CAD build for the part. Positions are in the model's coordinates, mm. Coordinates: 2 decimals unless noted, no trailing zeros. Order: outer loops, then holes, each group sorted by start corner. A loop starts at its lowest first (then second) coordinate and runs counter-clockwise, first axis right, second up. Notation, with made-up numbers: M 69.5,-3.5 L 74.5,-3.5 A18 cw 74.5,5.5 Z; hole C -6,35 d1. An arc over 180 degrees is marked long. One line per item, written item: value.
from build123d import *

# Parameters (mm, degrees)
F1_DEPTH = 38.1
F2_R     = 25.4
F2_R_2   = 2.413
F3_DEPTH = 25.4
F4_R     = 3.429
F5_DEPTH = 25.4


with BuildPart() as f1:
    # F0 (on Right) → F1 (new body, symmetric)
    with BuildSketch(Plane.YZ):
        with BuildLine():
            ThreePointArc((5.6640261054, -4.752682216), (1.7239069957, -3.6969304825), (0, 0))
            Line((0, 0), (0, 76.2))
            Line((0, 76.2), (-3.175, 76.2))
            Line((-3.175, 76.2), (-3.175, 0))
            ThreePointArc((-3.175, 0), (-0.3169436651, -6.1291215894), (6.2153590695, -7.8794468319))
            Line((6.2153590695, -7.8794468319), (35.9767941298, -2.6317028461))
            Line((35.9767941298, -2.6317028461), (35.4254611657, 0.4950617697))
            Line((35.4254611657, 0.4950617697), (5.6640261054, -4.752682216))
        make_face()
    extrude(amount=F1_DEPTH, both=True)

    # F2 (on face) → F3 (cut)
    with BuildSketch(Plane.XZ.offset(3.175)):
        with Locations((0, 38.1)):
            Circle(F2_R)
        with Locations((-26.8363952125, 22.606)):
            Circle(F2_R_2)
        with Locations((0, 69.088)):
            Circle(F2_R_2)
        with Locations((26.8363952125, 22.606)):
            Circle(F2_R_2)
    extrude(amount=-F3_DEPTH, mode=Mode.SUBTRACT)

    # F4 (on face) → F5 (cut)
    with BuildSketch(Plane(origin=(0, 0.9835478115, -5.5779768219), x_dir=(1, 0, 0), z_dir=(0, -0.1736481777, 0.984807753))):
        with Locations((19.05, 15.9232353842)):
            Circle(F4_R)
        with Locations((-19.05, 15.9232353842)):
            Circle(F4_R)
    extrude(amount=-F5_DEPTH, mode=Mode.SUBTRACT)


solid = f1.part
Q1. Pin check, flat tips, straight feed: pin 1 Ø6 at (x, y) = (29.5, 13.5) entering from -Z; pin 2 Ø5.5 at (x, z) = (-26.84, 22.61) entering from +Y; pin 3 Ø4 at (x, z) = (0, 69.088) entering from -Y; pin 4 Ø1.5 at (x, y) = (-3.5, 9) entering from -Z. Stop position of each tip, or through.
Recorded:
pin 1: stops at z = -7.12
pin 2: stops at y = 0
pin 3: passes through
pin 4: stops at z = -7.52
Q2. Mould opens along Y. For faces 1 (the face through (38.1, -1, 22)), 2 (the face through (0.533, 1.769, -3.735)), 3 (the face through (0.533, 20.753, -2.092)), 4 (the face through (1, -3.175, 64)) say: released by +Y, released by -Y, zero draft, split by the parting line, or undercut.
Recorded:
face 1: zero draft
face 2: undercut
face 3: undercut
face 4: released by -Y
Q3. Slice it at A-A (z = 38.1). List the corners of the cut face in (x, y) (3 decimals).
Recorded:
outline: M -38.1,-3.175 L -25.4,-3.175 L -25.4,0 L -38.1,0 Z; M 25.4,-3.175 L 38.1,-3.175 L 38.1,0 L 25.4,0 Z
Q4. Slice it at D-D (x = -19). List the corners of the cut face in (y, z) (3 decimals), plus the area to 3 significant figures.
Recorded:
outline: M -3.175,0 A8.001 ccw 6.215,-7.879 L 13.84,-6.535 L 13.288,-3.408 L 5.664,-4.753 A4.826 cw 0,0 L 0,21.243 L -3.175,21.243 Z; M -3.175,54.957 L 0,54.957 L 0,76.2 L -3.175,76.2 Z; M 20.041,-2.218 L 20.593,-5.344 L 35.977,-2.632 L 35.425,0.495 Z
area: 245 mm^2
Q5. Drill centre lines: line 1 along Z through (x, y) = (0, -1.5) (3 decimals); line 2 along X through (y, z) = (-2, 38); line 3 along Y through (x, z) = (23.5, 52.5) (3 decimals). Where is each one in solid material? Low to high.
Recorded:
line 1: z = -4.899 to 12.7, 63.5 to 66.675, 71.501 to 76.2
line 2: x = -38.1 to -25.4, 25.4 to 38.1
line 3: y = -3.175 to 0
Q6. Slice it at B-B (x = 0). List the corners of the cut face in (y, z) (3 decimals).
Recorded:
outline: M -3.175,0 A8.001 ccw 6.215,-7.879 L 35.977,-2.632 L 35.425,0.495 L 5.664,-4.753 A4.826 cw 0,0 L 0,12.7 L -3.175,12.7 Z; M -3.175,63.5 L 0,63.5 L 0,66.675 L -3.175,66.675 Z; M -3.175,71.501 L 0,71.501 L 0,76.2 L -3.175,76.2 Z
Q7. Slice it at C-C (x = -9.5). List the corners of the cut face in (y, z) (3 decimals), plus the area to 3 significant figures.
Recorded:
outline: M -3.175,0 A8.001 ccw 6.215,-7.879 L 35.977,-2.632 L 35.425,0.495 L 5.664,-4.753 A4.826 cw 0,0 L 0,14.543 L -3.175,14.543 Z; M -3.175,61.657 L 0,61.657 L 0,76.2 L -3.175,76.2 Z
area: 224 mm^2
